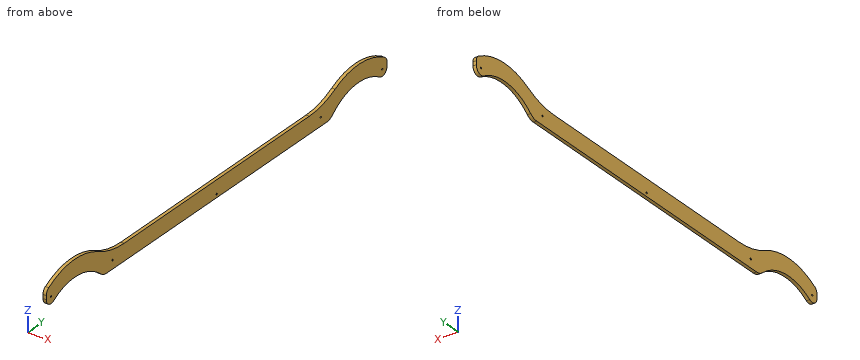
from build123d import *

# Parameters (mm, degrees)
F1_DEPTH      = 12.7
F2_R          = 3.175
F3_DEPTH      = 25.4
F3_DEPTH_BACK = 1882


# Not quite as in the source:
# - an extrude ends at something that could not be found from the text; its depth is read off the source's solid


with BuildPart() as f1:
    # F0 (on Right) → F1 (new body)
    with BuildSketch(Plane.YZ):
        with BuildLine():
            ThreePointArc((-622.6993794949, 12.1531100478), (-607.2983658108, 3.1350127999), (-589.7288184286, 0))
            Line((-589.7288184286, 0), (589.7288184286, 0))
            ThreePointArc((589.7288184286, 0), (607.2983658108, 3.1350127999), (622.6993794949, 12.1531100478))
            ThreePointArc((622.6993794949, 12.1531100478), (746.0500791914, 62.9065317561), (875.5608465608, 30.9962502452))
            ThreePointArc((875.5608465608, 30.9962502452), (901.3248834202, 30.3402571366), (914.4, 52.5496526411))
            Line((914.4, 52.5496526411), (914.4, 67.3727526142))
            ThreePointArc((914.4, 67.3727526142), (911.0154605337, 80.0408028781), (901.7638190955, 89.3328282539))
            ThreePointArc((901.7638190955, 89.3328282539), (769.7029358002, 126.8933113968), (635.7649329622, 96.7026143791))
            ThreePointArc((635.7649329622, 96.7026143791), (568.5593617374, 71.9168669296), (497.4251334688, 63.5))
            Line((497.4251334688, 63.5), (-497.4251334688, 63.5))
            ThreePointArc((-497.4251334688, 63.5), (-568.5593617374, 71.9168669296), (-635.7649329622, 96.7026143791))
            ThreePointArc((-635.7649329622, 96.7026143791), (-769.7029358002, 126.8933113968), (-901.7638190955, 89.3328282539))
            ThreePointArc((-901.7638190955, 89.3328282539), (-911.0154605337, 80.0408028781), (-914.4, 67.3727526142))
            Line((-914.4, 67.3727526142), (-914.4, 52.5496526411))
            ThreePointArc((-914.4, 52.5496526411), (-901.3248834202, 30.3402571366), (-875.5608465608, 30.9962502452))
            ThreePointArc((-875.5608465608, 30.9962502452), (-746.0500791914, 62.9065317561), (-622.6993794949, 12.1531100478))
        make_face()
    extrude(amount=F1_DEPTH)

    # F2 (on face) → F3 (cut, two sides)
    with BuildSketch(Plane.YZ.offset(12.7)) as f3_sk:
        with Locations((-889, 52.5496526411)):
            Circle(F2_R)
        with Locations((-558.8, 31.75)):
            Circle(F2_R)
        with Locations((0, 12.7)):
            Circle(F2_R)
        with Locations((558.8, 31.75)):
            Circle(F2_R)
        with Locations((889, 52.5496526411)):
            Circle(F2_R)
    extrude(amount=-F3_DEPTH, mode=Mode.SUBTRACT)
    extrude(f3_sk.sketch, amount=F3_DEPTH_BACK, mode=Mode.SUBTRACT)


solid = f1.part
Input: part model. Units: mm. Frame: model coordinates. Give positions to 0.01 mm unless a question says otherwise; leave off trailing zeros. Write each loop counter-clockwise with the first axis right and the second up, starting at its lowest first coordinate (ties: lowest second). Pieces come first, ordered by that corner, then holes.
Q1. Section B-B, the plane y = -171.5. Output: boundary loops of the cut face in (x, z), plus the area to 3 significant figures.
Q2. Section A-A, the plane x = 10.25. Output: boundary loops of the cut face in (y, z) (3 decimals).
Q3. Section C-C, the plane y = -517.5. Output: boundary loops of the cut face in (x, z), plus the area to 3 significant figures.
Q4. Material intervals for probe 1 along Y at (x, z) = (3.25, 41); probe 2 along Z at (x, y) = (4.75, -31.5); probe 3 along Y at (x, z) = (8, 44.5), sorted ascending.
Q5. First-contact query: P1, Ø1, axis at x = 8.5, z = 76, coming from the -Y side; P2, Ø1, axis at x = 5.5, y = 107, coming from the +Z side. Flat tips, straight axial feed; report the tip coordinate or a pass-through.
Filled in:
1. outline: (0, 0) - (12.7, 0) - (12.7, 63.5) - (0, 63.5) - close
1. area: 806 mm2
2. outline: (-914.4, 52.55) arc R25.4 ccw to (-875.561, 30.996) arc R214.63 cw to (-622.699, 12.153) arc R50.8 ccw to (-589.729, 0) - (589.729, 0) arc R50.8 ccw to (622.699, 12.153) arc R214.63 cw to (875.561, 30.996) arc R25.4 ccw to (914.4, 52.55) - (914.4, 67.373) arc R25.4 ccw to (901.764, 89.333) arc R278.13 ccw to (635.765, 96.703) arc R304.8 cw to (497.425, 63.5) - (-497.425, 63.5) arc R304.8 cw to (-635.765, 96.703) arc R278.13 ccw to (-901.764, 89.333) arc R25.4 ccw to (-914.4, 67.373) - close; hole circle Ø6.35 at (-889, 52.55); hole circle Ø6.35 at (-558.8, 31.75); hole circle Ø6.35 at (0, 12.7); hole circle Ø6.35 at (558.8, 31.75); hole circle Ø6.35 at (889, 52.55)
3. outline: (0, 0) - (12.7, 0) - (12.7, 64.16) - (0, 64.16) - close
3. area: 815 mm2
4. probe 1: y = -911.62 to -857.67, -666.33 to 666.33, 857.67 to 911.62
4. probe 2: z = 0 to 63.5
4. probe 3: y = -913.09 to -850.29, -673.71 to 673.71, 850.29 to 913.09
5. P1: stops at y = -913.06
5. P2: stops at z = 63.5
